Geometry: see drawing. Coordinates: mm, zero at the bounding-box minimum. Give positions to 0.01 mm unless a question says otherwise; leave off trailing zeros. Write each loop counter-clockwise with the first axis right and the second up, starting at its lowest first coordinate (ties: lowest second). Pieces come first, ordered by that corner, then holes. Notation, with made-up numbers: (-23, -13.75) -> (34, -13.75) arc R20 ccw to (34, 14.25) -> close; hole circle Ø1 at (21, -14.5). An arc over 180 degrees is marked (long way). Use one line per item in the form item = value. Start each with the question number.
(1) Cut plane A-A, the plane x = 30. Output: boundary loops of the cut face in (y, z), and give its area (3 significant figures).
(2) Cut plane B-B, the plane z = 4.25. Output: boundary loops of the cut face in (x, y).
(3) Draft query along X for the marked faces 1 and 2. Return one class per face: pulls with the +X half, pulls with the -X half, needs draft (parallel to the pull), parting line crosses it, or undercut.
(4) Cut plane C-C, the plane x = 95.5. Output: boundary loops of the cut face in (y, z).
(5) First-contact query: P1, Ø2, axis at y = 4.5, z = 1, coming from the -X side; P2, Ø12, axis at x = 18, y = 8.5, coming from the +Z side; P3, Ø6, axis at y = 16.5, z = 7, coming from the +X side. Flat tips, straight axial feed; report the tip coordinate or a pass-through.
(6) Material intervals for line 1 along X through (y, z) = (17, 2.75); line 2 along Y through (x, z) = (95, 7); line 3 along Z through (x, y) = (76, 19.5), sorted ascending. Write a range as from..to.
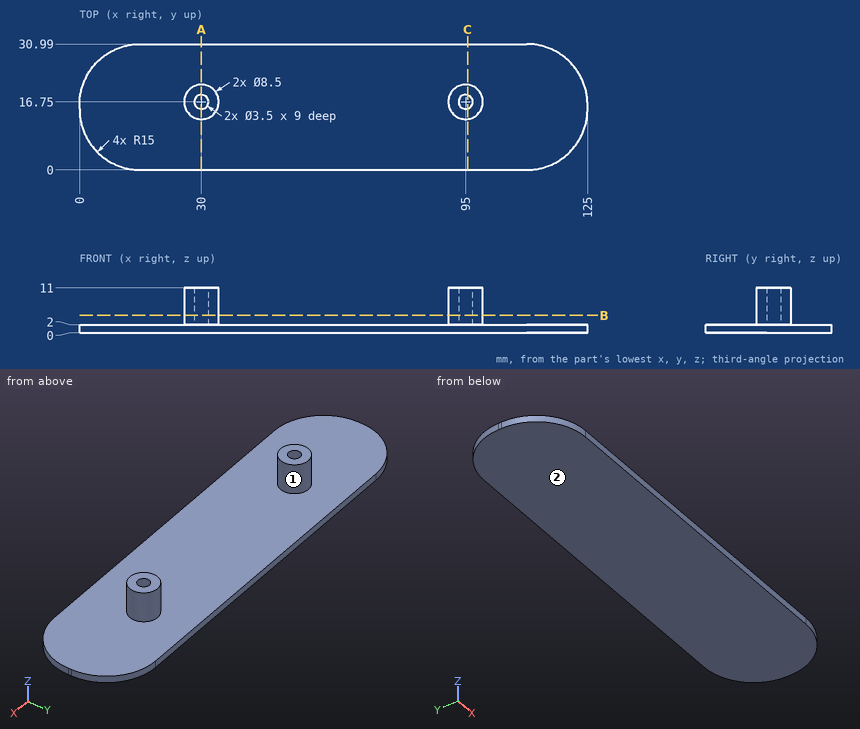
Geometry says:
q1.outline = (0, 0) -> (30.99, 0) -> (30.99, 2) -> (21, 2) -> (21, 11) -> (18.5, 11) -> (18.5, 2) -> (15, 2) -> (15, 11) -> (12.5, 11) -> (12.5, 2) -> (0, 2) -> close
q1.area = 107 mm^2
q2.outline = circle Ø8.5 at (30, 16.75); circle Ø8.5 at (95, 16.75); hole circle Ø3.5 at (30, 16.75); hole circle Ø3.5 at (95, 16.75)
q3.face_1 = undercut
q3.face_2 = needs draft
q4.outline = (0, 0) -> (30.99, 0) -> (30.99, 2) -> (20.97, 2) -> (20.97, 11) -> (18.43, 11) -> (18.43, 2) -> (15.07, 2) -> (15.07, 11) -> (12.53, 11) -> (12.53, 2) -> (0, 2) -> close
q5.P1 = 3.39
q5.P2 = 2
q5.P3 = 99.25
q6.line_1 = 25.76..28.27, 31.73..34.24, 90.76..93.27, 96.73..99.24
q6.line_2 = 12.5..15, 18.5..21
q6.line_3 = 0..2
